Can you work these out from the drawing? Everything is in mm from the part's minimum corner. Round coordinates to 2 decimals unless told otherwise and drop trailing zeros. Loops run counter-clockwise (first coordinate to the right, second up) from the corner with the lowest first, then second, coordinate; pieces in that order, holes last. Notation, with made-up numbers: M 35,85.25 L 51,85.25 A6 cw 51,94.25 Z; hole C 26,58 d11. An arc over 180 degrees is marked long. Answer in a Markdown table with one row per item.
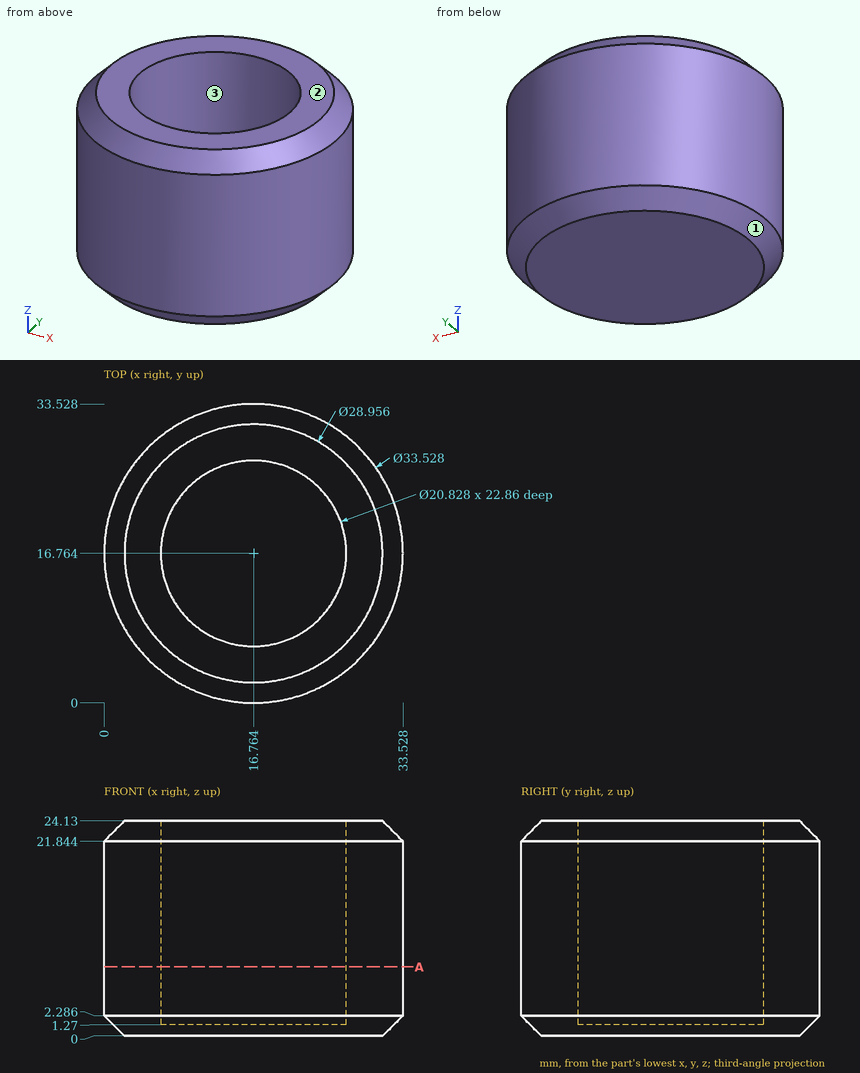
1) I need wall thicknesses on line 1 (Z direction, x = 17, y = 20); line 2 (Y direction, x = 22, z = 7); line 3 (Y direction, x = 10.5, z = 12). Which ranges of each line are inside material? Lowest first, please.
Computed:
| item | result |
|---|---|
| line 1 | z = 0 to 1.27 |
| line 2 | y = 0.84 to 7.76, 25.77 to 32.69 |
| line 3 | y = 1.21 to 8.44, 25.08 to 32.31 |
2) Will these pins go through, and if not, where does the flat tip stop? P1, Ø16.5, axis at x = 19.5, y = 15.5, coming from the +Z side; P2, Ø1, axis at x = 18.5, z = 14, coming from the +Y side; P3, Ø2, axis at x = 11, z = 18.5, coming from the +Y side; P4, Ø5, axis at y = 29.5, z = 12, coming from the -X side.
Computed:
| item | result |
|---|---|
| P1 | stops at z = 24.13 |
| P2 | stops at y = 33.48 |
| P3 | stops at y = 32.84 |
| P4 | stops at x = 3.49 |
3) I want a section at A-A, the plane z = 7.75. Please give me the cut outline in (x, y).
Computed:
| item | result |
|---|---|
| outline | C 16.76,16.76 d33.53; hole C 16.76,16.76 d20.83 |
4) If we mould it in two halves opening along Y, with no side actions, what happens to the marked faces 1, 2 and 3? For each: released by +Y, released by -Y, zero draft, split by the parting line, or undercut.
Computed:
| item | result |
|---|---|
| face 1 | split by the parting line |
| face 2 | zero draft |
| face 3 | undercut |
